For this review, take the finished solid that the model builds, in its own axes (mm). A direction names the side the tool comes from. Give positions to 0.01 mm unless a question says otherwise; leave off trailing zeros. Loops run counter-clockwise (first coordinate to the right, second up) from the corner with the lowest first, then second, coordinate; pieces in that order, holes last. Notation, with made-up numbers: M 6,70 L 14,70 A8 cw 14,75 Z; hole C 10.5,-36.5 d9. An arc over 180 degrees is marked long. Use CSV: the item, a comma, the result in double quotes. Start each with the question number.
1. Insertion check: P1, Ø0.8, axis at y = -0.5, z = 21.5, coming from the +X side; P2, Ø1.1, axis at y = -1.5, z = 11, coming from the -X side; P3, Ø0.5, axis at y = -1.5, z = 15.5, coming from the +X side. Each pin has a flat end and moves straight along its axis. Give the tip position at first contact, or say it passes through.
2. Take a section at C-C, the plane x = -32.5. Write out the cut boundary in (y, z).
3. Take a section at A-A, the plane y = 7. Write out the cut boundary in (x, z), and give its area (3 significant figures).
4. Take a section at B-B, the plane z = 30.5. Write out the cut boundary in (x, y).
5. Take a section at D-D, the plane z = 44. Write out the cut boundary in (x, y), and give its area (3 significant figures).
6. To check wall thickness, follow line 1 (X direction, y = 11.5, z = 40.5); line 2 (Z direction, x = -15.5, y = 3.5); line 3 (X direction, y = -0.5, z = 8). State the ranges of each line that lie inside material, in increasing order. Write a range as [from, to].
7. The part is to be moulded in two halves that separate along X. For faces 4 (the face through (-53, -2, 19)), 5 (the face through (0, 8, 35)), 6 (the face through (-10, -1, 19)), say which applies: pulls with the +X half, pulls with the -X half, needs draft (parallel to the pull), parting line crosses it, or undercut.
8. Tool access review of faces 1 (the face through (-31, 9, 68)), 2 (the face through (-53, -1, 39)), 3 (the face through (-55, -1, 19)): name each direction out of +Z, -Z, +X, -X, +Y, -Y from which nothing blocks a thin tool from reaching the whole face with its end or side.
Autodesk Inventor part; units mm, degrees
ref_plane "YZ Plane" through (0, 0, 0) normal (1, 0, 0) x (0, 1, 0)
ref_plane "XZ Plane" through (0, 0, 0) normal (0, 1, 0) x (-1, 0, 0)
ref_plane "XY Plane" through (0, 0, 0) normal (0, 0, 1) x (1, 0, 0)
sketch "Sketch1" plane through (0, 0, 0) normal (0, 1, 0) x (-1, 0, 0)
  line L0 (0, 0) -> (62, 0)
  line L1 (62, 0) -> (62, 70)
  line L2 (62, 70) -> (0, 70)
  line L3 (0, 70) -> (0, 0)
  dimension "d0" = 62
  dimension "d1" = 70
extrude "Extrusion1" add sketch "Sketch1" along normal blind 2
sketch "Sketch2" plane through (0, 2, 0) normal (0, 1, 0) x (1, 0, 0)
  line L0 (0, 0) -> (-62, 0)
  line L1 (-62, 0) -> (-62, -70)
  line L2 (-62, -70) -> (0, -70)
  line L3 (0, -70) -> (0, 0)
  line L4 (-60, -2) -> (-2, -2)
  line L5 (-2, -2) -> (-2, -68)
  line L6 (-2, -68) -> (-60, -68)
  line L7 (-60, -68) -> (-60, -2)
  line L8 (0, 0) -> (-62, 0)
  line L9 (-62, 0) -> (-62, -70)
  line L10 (-62, -70) -> (0, -70)
  line L11 (0, -70) -> (0, 0)
  dimension "d4" = 2
  dimension "d5" = 2
  dimension "d6" = 2
  dimension "d7" = 2
extrude "Extrusion2" add sketch "Sketch2" along normal blind 15
fillet "Fillet1" radius 2 4 edges at (-62, 8.5, 70) (-62, 8.5, 0) (0, 8.5, 0) (0, 8.5, 70)
sketch "Sketch3" plane through (-2, 0, 0) normal (0, 0, -1) x (-1, 0, 0)
  line L0 (0, 0) -> (58, 0)
  line L1 (8.7434, -1) -> (3.7434, -1)
  line L2 (3.7434, -1) -> (3.7434, -2)
  line L3 (3.7434, -2) -> (8.7434, -2)
  line L4 (8.7434, -2) -> (8.7434, -1)
  line L5 (5.7434, 0) -> (6.7434, 0)
  line L6 (6.7434, 0) -> (6.7434, -1)
  line L7 (6.7434, -1) -> (5.7434, -1)
  line L8 (5.7434, -1) -> (5.7434, 0)
  line L9 (50.59, 0) -> (51.59, 0)
  line L10 (51.59, 0) -> (51.59, -1)
  line L11 (51.59, -1) -> (50.59, -1)
  line L12 (50.59, -1) -> (50.59, 0)
  line L13 (48.59, -1) -> (53.59, -1)
  line L14 (53.59, -1) -> (53.59, -2)
  line L15 (53.59, -2) -> (48.59, -2)
  line L16 (48.59, -2) -> (48.59, -1)
  point P0 (-2, 0)
  point P1 (29, 0)
  point P2 (9.41, 0)
  point P3 (48.59, 0)
  dimension "d11" = 19.59
  dimension "d12" = 19.59
  dimension "d14" = 2
  dimension "d15" = 2
  dimension "d16" = 2
  dimension "d17" = 2
  dimension "d18" = 2
  dimension "d19" = 1
  dimension "d20" = 1
  dimension "d21" = 1
  dimension "d22" = 1
  dimension "d23" = 1
  dimension "d24" = 1
extrude "Extrusion3" add sketch "Sketch3" against normal blind 39
properties part number "Insert"
Result set:
1,P1,"x = -7.74"
1,P2,"x = -55.59"
1,P3,"x = -5.74"
2,outline,"M 0,0 L 17,0 L 17,2 L 2,2 L 2,68 L 17,68 L 17,70 L 0,70 Z"
3,outline,"M -62,2 A2 ccw -60,0 L -2,0 A2 ccw 0,2 L 0,68 A2 ccw -2,70 L -60,70 A2 ccw -62,68 Z; hole M -60,2 L -2,2 L -2,68 L -60,68 Z"
3,area,"509 mm2"
4,outline,"M -62,0 L -53.59,0 L -53.59,-1 L -55.59,-1 L -55.59,-2 L -50.59,-2 L -50.59,-1 L -52.59,-1 L -52.59,0 L -8.74,0 L -8.74,-1 L -10.74,-1 L -10.74,-2 L -5.74,-2 L -5.74,-1 L -7.74,-1 L -7.74,0 L 0,0 L 0,17 L -2,17 L -2,2 L -60,2 L -60,17 L -62,17 Z"
5,outline,"M -62,0 L 0,0 L 0,17 L -2,17 L -2,2 L -60,2 L -60,17 L -62,17 Z"
5,area,"184 mm2"
6,line 1,"[-62, -60], [-2, 0]"
6,line 2,"[0, 2], [68, 70]"
6,line 3,"[-53.59, -52.59], [-8.74, -7.74]"
7,face 4,"needs draft"
7,face 5,"pulls with the +X half"
7,face 6,"undercut"
8,face 1,"+Y"
8,face 2,"+Z, +X, -X, -Y"
8,face 3,"+Z, -Z, -X"
